Source: CAD feature listing. Evaluate the final solid. Frame: model axes, mm. Coordinates: 2 decimals unless noted, no trailing zeros. Order: outer loops, then holes, each group sorted by start corner. A loop starts at its lowest first (then second) coordinate and runs counter-clockwise, first axis right, second up. Notation, with made-up numbers: (13, 41) -> (46, 41) arc R22 cw to (46, 78) -> close; hole circle Ø3 at (-29, -34.75). An arc over 180 degrees is marked (long way). Write item = value, one per line. Start each with the question number.
Item 1: Section query C-C (y = -94.5). Output: boundary loops of the cut face in (x, z), then the cut area to 3 significant figures.
Item 2: Section query A-A (y = -25.5). Output: boundary loops of the cut face in (x, z).
Item 3: Ray query, line 1 along Y through (x, z) = (0.75, 5.25); line 2 along Z through (x, y) = (-4, -37); line 3 along Z through (x, y) = (8.5, -30.5). Return the intervals inside material, ascending. Write a range as [from, to].
Item 4: Section query B-B (x = 2.25). Output: boundary loops of the cut face in (y, z).
Item 5: Contact query for flat-ended pins moving along their axis: pin 1 (12 mm diameter, centred on y = -22, z = 7, fed in from -X); pin 2 (2 mm diameter, centred on x = 4.5, y = -110.5, fed in from -Z); pin 3 (5 mm diameter, centred on x = -4.5, z = 2, fed in from -Y). Output: stop coordinate, or through.
```python
from build123d import *

# Parameters (mm, degrees)
F1_DEPTH = 130
F3_DEPTH = 12.5


with BuildPart() as f1:
    # F0 (on Front) → F1 (new body)
    with BuildSketch(Plane.XZ):
        Polygon((0, 10.606602), (-10.606602, 0), (0, -10.606602), (10.606602, 0), align=None)
    extrude(amount=F1_DEPTH)

    # F2 (on Right) → F3 (cut, symmetric)
    with BuildSketch(Plane.YZ):
        Polygon((-130, 10.815689), (-130, -10.600555), (-92.905977, 10.815689), align=None)
    extrude(amount=F3_DEPTH, both=True, mode=Mode.SUBTRACT)


solid = f1.part
```
Computed:
q1.outline = (-10.61, 0) -> (0, -10.61) -> (10.61, 0) -> (0.71, 9.9) -> (-0.71, 9.9) -> close
q1.area = 224 mm^2
q2.outline = (-10.61, 0) -> (0, -10.61) -> (10.61, 0) -> (0, 10.61) -> close
q3.line_1 = [-102.55, 0]
q3.line_2 = [-6.61, 6.61]
q3.line_3 = [-2.11, 2.11]
q4.outline = (-126.11, -8.36) -> (0, -8.36) -> (0, 8.36) -> (-97.17, 8.36) -> close
q5.pin_1 = -9.61
q5.pin_2 = -7.11
q5.pin_3 = -112.51
